```python
from build123d import *

# Parameters (mm, degrees)
EXTRUSION1_DEPTH   = 30
FILLET1_R          = 3.175
SKETCH2_R          = 1
EXTRUSION8_DEPTH   = 2
SKETCH3_R          = 2.15
EXTRUSION11_DEPTH  = 71.357498555
EXTRUSION12_DEPTH  = 9.525
CUT_EXTRUDE1_DEPTH = 1.27


with BuildPart() as part:
    # Sketch1 → Extrusion1 (new body)
    with BuildSketch(Plane.XY):
        with BuildLine():
            Line((47.06353616, 19.123444108), (42.213867638, 19.070033288))
            ThreePointArc((42.213867638, 19.070033288), (46.321150196, -0.088533061), (42.140232503, -19.23116511))
            Line((42.140232503, -19.23116511), (27.063632515, -19.23116511))
            Line((27.063632515, -19.23116511), (27.063633082, -22.12345478))
            Line((27.063633082, -22.12345478), (27.063633082, -23.62345478))
            Line((27.063633082, -23.62345478), (44.972996835, -23.62345478))
            ThreePointArc((44.972996835, -23.62345478), (49.168432062, -12.771632691), (50.784831526, -1.249871881))
            Line((50.784831526, -1.249871881), (48.284855505, -1.250061095))
            Line((48.284855505, -1.250061095), (48.284855505, 1.249938905))
            Line((48.284855505, 1.249938905), (50.784855505, 1.249938905))
            ThreePointArc((50.784855505, 1.249938905), (49.733715684, 10.355236056), (47.06353616, 19.123444108))
        make_face()
    extrude(amount=EXTRUSION1_DEPTH)

    # Fillet1
    fillet1_edges = [part.edges().sort_by_distance(p)[0] for p in [
        (42.140232503, -19.23116511, 15),
    ]]
    fillet(fillet1_edges, radius=FILLET1_R)

    # Sketch2 → Extrusion8 (cut)
    with BuildSketch(Plane(origin=(48.284855505, 0, 0), x_dir=(0, 0, -1), z_dir=(1, 0, 0))):
        with Locations(Location((-24, -6.1095e-05, 0), (0, 0, 90))):
            Circle(SKETCH2_R)
        with Locations(Location((-6, -6.1095e-05, 0), (0, 0, 90))):
            Circle(SKETCH2_R)
    extrude(amount=-EXTRUSION8_DEPTH, mode=Mode.SUBTRACT)

    # Sketch3 → Extrusion11 (cut, through all)
    with BuildSketch(Plane(origin=(0, -19.23116511, 0), x_dir=(-1, 0, 0), z_dir=(0, 1, 0))):
        with Locations((-34.601932509, 8)):
            Circle(SKETCH3_R)
        with Locations((-34.601932509, 22)):
            Circle(SKETCH3_R)
    extrude(amount=-EXTRUSION11_DEPTH, mode=Mode.SUBTRACT)

    # Sketch4 → Extrusion12 (cut, symmetric)
    with BuildSketch(Plane.XY.offset(15)):
        with BuildLine():
            Line((49.784318727, 1.249938905), (50.784855505, 1.249938905))
            ThreePointArc((50.784855505, 1.249938905), (49.733715684, 10.355236056), (47.06353616, 19.123444108))
            Line((47.06353616, 19.123444108), (45.987026195, 19.111588188))
            ThreePointArc((45.987026195, 19.111588188), (48.711366707, 10.356301793), (49.784318727, 1.249938905))
        make_face()
        with BuildLine():
            ThreePointArc((44.364346419, -22.62345478), (48.272126893, -12.240444134), (49.784292363, -1.249947608))
            Line((49.784292363, -1.249947608), (50.784831526, -1.249871881))
            ThreePointArc((50.784831526, -1.249871881), (49.168432062, -12.771632691), (44.972996835, -23.62345478))
            Line((44.972996835, -23.62345478), (27.063633082, -23.62345478))
            Line((27.063633082, -23.62345478), (27.063633082, -22.62345478))
            Line((27.063633082, -22.62345478), (44.364346419, -22.62345478))
        make_face()
    extrude(amount=EXTRUSION12_DEPTH, both=True, mode=Mode.SUBTRACT)

    # Sketch5 → Cut-Extrude1 (cut)
    with BuildSketch(Plane.ZY.offset(-27.063633082)):
        Polygon((0, -19.23116511), (0, -23.62345478), (5.475, -23.62345478), (5.475, -22.62345478), (24.525, -22.62345478), (24.525, -23.62345478), (30, -23.62345478), (30, -19.23116511), align=None)
    extrude(amount=-CUT_EXTRUDE1_DEPTH, mode=Mode.SUBTRACT)


with BuildPart() as cut_extrude1_kept_piece:
    # of the separate pieces the step leaves, the one the design keeps (cut_extrude1_pieces_kept)
    add(part.part.solids().sort_by_distance((42.99418243, -17.237727528, 0))[0])


solid = cut_extrude1_kept_piece.part
```
For this review, take the finished solid that the model builds, in its own axes (mm). A direction names the side the tool comes from. Coordinates: 2 decimals unless noted, no trailing zeros. Loops run counter-clockwise (first coordinate to the right, second up) from the corner with the lowest first, then second, coordinate; pieces in that order, holes last.
1. For line 1 (Y direction, x = 30.5, z = 21); line 2 (X direction, y = 1, z = 10.5); line 3 (Y direction, x = 30, z = 25), list the stretches that pass through material, from the lowest coordinate up.
2. Mouldability with a two-part tool opening along X and no side actions: class faces 4 (the flat face through (46, -7, 0)), 5 (the cylindrical face through (49.76, 10.23, 27.22)), 6 (the cylindrical face through (36.308, -20.904, 20.692)) as +X half, -X half, draft (parallel to the pull), parting line (faces both ways), or undercut.
3. For faces 1 (the flat face through (49, 10, 24.525)), 2 (the cylindrical face through (48.234, -12.391, 15.133)), 3 (the flat face through (48.285, 0, 15)), list the 3-axis set-ups (+Z, -Z, +X, -X, +Y, -Y) from which the entire face can be reached by the end or side of a thin tool; tool diameter is ignored.
4. Add section B-B, the plane y = 0. Give the boundary of the cut face in (x, z).
5. Insertion check: P1, Ø1.5, axis at y = -14, z = 22.5, coming from the -X side; P2, Ø3, axis at y = -18, z = 25.5, coming from the +X side; P3, Ø2.5, axis at y = 0, z = 6, coming from the -X side; P4, Ø3.5, axis at x = 34.6, z = 22, coming from the -Y side. Each pin has a flat end and moves straight along its axis. Give the tip position at first contact, or say it passes through.
6. Add section A-A, the plane z = 22. Give the boundary of the cut face in (x, y) (3 decimals), then the cut area to 3 significant figures.
7. Add section C-C, the plane x = 34.75. Give the boundary of the cut face in (y, z) (3 decimals).
8. Add section D-D, the plane z = 28.5. Give the boundary of the cut face in (x, y) (3 decimals), then the cut area to 3 significant figures.
Result:
1. line 1: y = -22.62 to -19.23
1. line 2: x = 46.31 to 48.28
1. line 3: y = -23.62 to -19.23
2. face 4: draft
2. face 5: +X half
2. face 6: undercut
3. face 1: +X, +Y
3. face 2: +X, -Y
3. face 3: +Z, -Z, +X
4. outline: (46.32, 0) - (48.28, 0) - (48.28, 5) - (46.32, 5) - close; (46.32, 7) - (48.28, 7) - (48.28, 23) - (46.32, 23) - close; (46.32, 25) - (48.28, 25) - (48.28, 30) - (46.32, 30) - close
5. P1: stops at x = 43.91
5. P2: stops at x = 48.05
5. P3: stops at x = 46.3
5. P4: passes through
6. outline: (28.334, -22.623) - (32.452, -22.623) - (32.452, -19.231) - (28.334, -19.231) - close; (36.752, -22.623) - (44.364, -22.623) arc R49.8 ccw to (49.784, -1.25) - (48.285, -1.25) - (48.285, 1.25) - (49.784, 1.25) arc R49.8 ccw to (45.987, 19.112) - (42.214, 19.07) arc R46.321 cw to (42.994, -17.238) arc R3.175 cw to (40.047, -19.231) - (36.752, -19.231) - close
6. area: 177 mm2
7. outline: (-23.623, 0) - (-19.231, 0) - (-19.231, 5.855) - (-22.623, 5.855) - (-22.623, 5.475) - (-23.623, 5.475) - close; (-23.623, 24.525) - (-22.623, 24.525) - (-22.623, 24.145) - (-19.231, 24.145) - (-19.231, 30) - (-23.623, 30) - close; (-22.623, 10.145) - (-19.231, 10.145) - (-19.231, 19.855) - (-22.623, 19.855) - close
8. outline: (28.334, -23.623) - (44.973, -23.623) arc R50.8 ccw to (50.785, -1.25) - (48.285, -1.25) - (48.285, 1.25) - (50.785, 1.25) arc R50.8 ccw to (47.064, 19.123) - (42.214, 19.07) arc R46.321 cw to (42.994, -17.238) arc R3.175 cw to (40.047, -19.231) - (28.334, -19.231) - close
8. area: 249 mm2
